For this review, take the finished solid that the model builds, in its own axes (mm). Face numbers are marked on the shaded views. Give positions to 0.01 mm unless a question says otherwise; leave off trailing zeros. Write each loop counter-clockwise with the first axis right and the second up, starting at its lowest first coordinate (ties: lowest second). Pieces come first, ordered by that corner, then holes.
Autodesk Inventor part; units mm, degrees
ref_plane "YZ Plane" through (0, 0, 0) normal (1, 0, 0) x (0, 1, 0)
ref_plane "XZ Plane" through (0, 0, 0) normal (0, 1, 0) x (-1, 0, 0)
ref_plane "XY Plane" through (0, 0, 0) normal (0, 0, 1) x (1, 0, 0)
sketch "Sketch2" plane through (0, 0, 0) normal (0, 0, 1) x (1, 0, 0)
  line L0 (0, 0) -> (18.2937, 0)
  line L1 (0, 4.2) -> (0, 7)
  line L2 (0, 7) -> (1.5, 7)
  line L3 (1.5, 7) -> (1.5, 6.5)
  line L4 (1.5, 6.5) -> (2.5, 6.5)
  line L5 (2.5, 6.5) -> (2.5, 7)
  line L6 (2.5, 7) -> (13, 7)
  line L7 (13, 7) -> (13, 4.2)
  line L8 (0, 4.2) -> (1, 3)
  line L9 (1, 3) -> (1, 0)
  line L10 (13, 4.2) -> (12, 3)
  line L11 (12, 3) -> (12, 0)
  dimension "d12" = 13
  dimension "d13" = 7
  dimension "d14" = 1.5
  dimension "d15" = 1
  dimension "d16" = 0.5
  dimension "d17" = 3
  dimension "d18" = 1
  dimension "d19" = 1.2
  dimension "d20" = 1
revolve "Revolution1" add sketch "Sketch2" angle 360 about axis through (0, 0, 0) along (1, 0, 0)
hole "Hole2" at (1, 0, 0) direction (1, 0, 0) diameter 4.917 end through all
properties part number "igus_DST-JSRM-1413DS6.35x2.54"
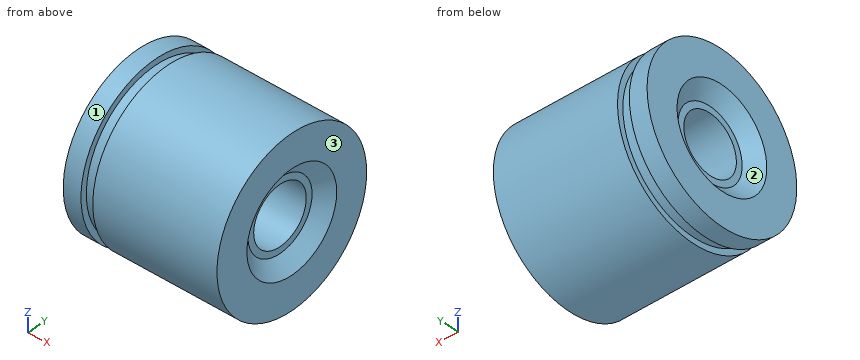
(1) The part is to be moulded in two halves that separate along Z. For the marked faces 1, 2 and 3, say which applies: +Z half, -Z half, draft (parallel to the pull), parting line (faces both ways), or undercut.
(2) We need section D-D (y = 4.5). Write out the cut boundary in (x, z), and give its area (3 significant figures).
(3) Clearance check with flat-ended pins moving along their axes: pin 1 Ø3 at (x, z) = (4.5, 2.5) entering from +Y; pin 2 Ø5 at (y, z) = (0.5, 1) entering from +X (3 decimals); pin 3 Ø2 at (y, z) = (2.5, -0.5) entering from -X; pin 4 Ø4 at (y, z) = (-0.5, -2.5) entering from -X. State where each tip first meets the part, or that it passes through.
(4) We need section A-A (z = 0). Write out the cut boundary in (x, y).
(5) For L1, parallel to Z at x = 6, y = 0; L2, parallel to X at y = -5.25, z = 4.25; L3, parallel to Y at x = 8.75, z = -1, list the stretches that pass through material, from the lowest coordinate up.
(6) We need section C-C (x = 4.25). Write out the cut boundary in (y, z), and give its area (3 significant figures).
The answers:
1. face 1: parting line
1. face 2: undercut
1. face 3: draft
2. outline: (0, -5.36) - (1.5, -5.36) - (1.5, -4.69) - (2.5, -4.69) - (2.5, -5.36) - (13, -5.36) - (13, 5.36) - (2.5, 5.36) - (2.5, 4.69) - (1.5, 4.69) - (1.5, 5.36) - (0, 5.36) - close
2. area: 138 mm2
3. pin 1: stops at y = 6.93
3. pin 2: stops at x = 12.515
3. pin 3: stops at x = 0.54
3. pin 4: stops at x = 0
4. outline: (0, -7) - (1.5, -7) - (1.5, -6.5) - (2.5, -6.5) - (2.5, -7) - (13, -7) - (13, -4.2) - (12, -3) - (12, -2.46) - (1, -2.46) - (1, -3) - (0, -4.2) - close; (0, 4.2) - (1, 3) - (1, 2.46) - (12, 2.46) - (12, 3) - (13, 4.2) - (13, 7) - (2.5, 7) - (2.5, 6.5) - (1.5, 6.5) - (1.5, 7) - (0, 7) - close
5. L1: z = -7 to -2.46, 2.46 to 7
5. L2: x = 0 to 1.5, 2.5 to 13
5. L3: y = -6.93 to -2.25, 2.25 to 6.93
6. outline: circle Ø14 at (0, 0); hole circle Ø4.92 at (0, 0)
6. area: 135 mm2
